Design review of the part shown in the three views and the two pictorial views. Dimensions are in mm from the part's minimum x, y and z. Coordinates: 2 decimals unless noted, no trailing zeros. Loops run counter-clockwise (first coordinate to the right, second up) from the corner with the lowest first, then second, coordinate; pieces in that order, holes last. Notation, with made-up numbers: M 84,-32.75 L 140,-32.75 A34 cw 140,6.25 Z; hole C 72.25,61.25 d3. An arc over 180 degrees is marked long. Answer as a JSON object with one key per item and string values. Group by question number.
Item 1: Mouldability with a two-part tool opening along X and no side actions: class the marked faces 1, 2 and 3 as +X half, -X half, draft (parallel to the pull), parting line (faces both ways), or undercut.
Item 2: Wall thickness on L1, parallel to Y at x = 7.5, z = 7; L2, parallel to Z at x = 6.5, y = 4.75; L3, parallel to X at y = 9, z = 9.5: over which ranges is each line inside the solid? List them lowest first. Write a range as from..to.
Item 3: Add section B-B (z = 6.5). State the section outline as (x, y) points, then the cut area to 3 significant figures.
Item 4: Insertion check: pin 1 (4 mm diameter, centred on y = 2, z = 4.5, fed in from +X); pin 2 (2 mm diameter, centred on x = 11.5, z = 11.5, fed in from +Y); pin 3 (4 mm diameter, centred on x = 13.5, z = 4.5, fed in from -Y). Each pin has a flat end and moves straight along its axis. Give the tip position at first contact, or say it passes through.
Item 5: Add section A-A (x = 7.5). State the section outline as (y, z) points.
Item 6: Add section C-C (z = 12.5). State the section outline as (x, y) points, then the cut area to 3 significant figures.
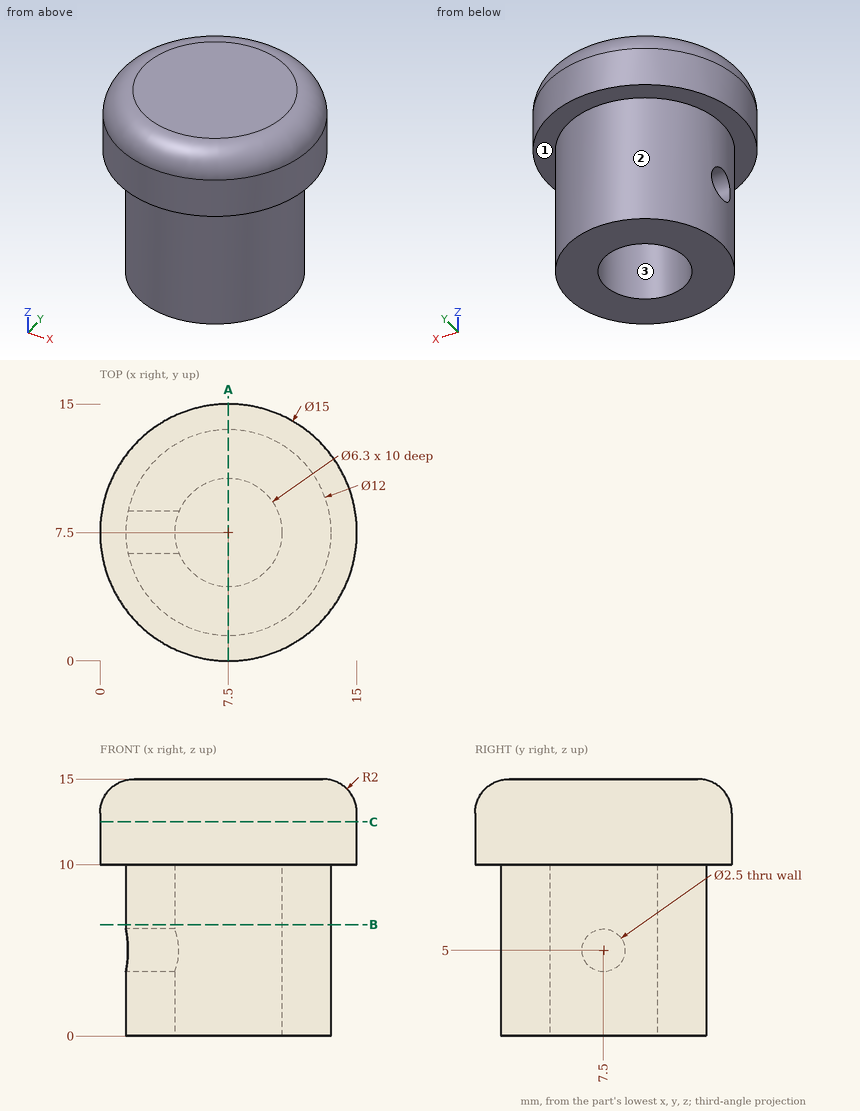
From the geometry:
{
 "1": {"face 1": "draft", "face 2": "parting line", "face 3": "undercut"},
 "2": {"L1": "y = 1.5..4.35, 10.65..13.5", "L2": "z = 10..15", "L3": "x = 1.69..4.73, 10.27..13.31"},
 "3": {"outline": "C 7.5,7.5 d12; hole C 7.5,7.5 d6.3", "area": "81.9 mm²"},
 "4": {"pin 1": "stops at x = 12.37", "pin 2": "stops at y = 14.37", "pin 3": "stops at y = 3.03"},
 "5": {"outline": "M 0,10 L 1.5,10 L 1.5,0 L 4.35,0 L 4.35,10 L 10.65,10 L 10.65,0 L 13.5,0 L 13.5,10 L 15,10 L 15,13 A2 ccw 13,15 L 2,15 A2 ccw 0,13 Z"},
 "6": {"outline": "C 7.5,7.5 d15", "area": "177 mm²"}
}
